Model file for the job. Use its own axes, mm. Round coordinates to 2 decimals unless told otherwise and drop trailing zeros. Write each loop counter-clockwise with the first axis right and the second up, starting at its lowest first coordinate (ties: lowest second). Pieces come first, ordered by that corner, then holes. Notation, with made-up numbers: (-10, 21) - (35, 21) arc R24 cw to (35, 43) - close; hole circle Ø5 at (60, -28). An arc over 180 degrees is marked (long way). One line per item, written item: value.
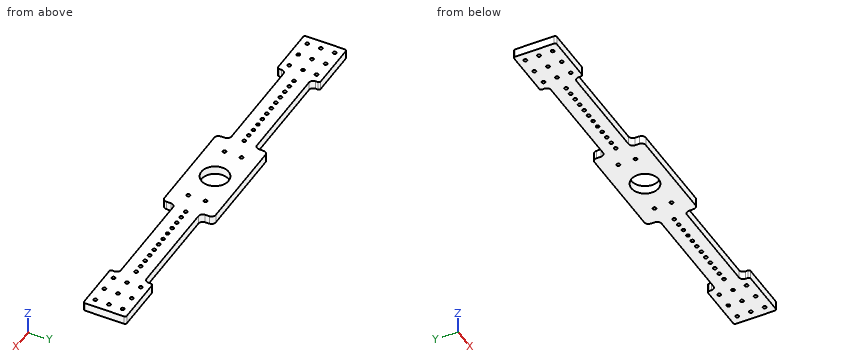
from build123d import *

# Parameters (mm, degrees)
BOSS_EXTRUDE1_DEPTH = 10
SKETCH2_R           = 2
SKETCH2_R_2         = 16
CUT_EXTRUDE1_DEPTH  = 11
FILLET1_R           = 5
SKETCH3_R           = 2
CUT_EXTRUDE2_DEPTH  = 11
SKETCH4_R           = 2
CUT_EXTRUDE3_DEPTH  = 11
LPATTERN1_COUNT     = 6
LPATTERN1_PITCH     = 10
LPATTERN1_COL_COUNT = 6
LPATTERN1_COL_PITCH = 10
SKETCH5_R           = 2
CUT_EXTRUDE4_DEPTH  = 11
FILLET2_R           = 2


with BuildPart() as part:
    # Sketch1 → Boss-Extrude1 (new body)
    with BuildSketch(Plane.XY):
        Polygon((245, 5), (245, 55), (185, 55), (185, 45), (60, 45), (60, 60), (-60, 60), (-60, 45), (-185, 45), (-185, 55), (-245, 55), (-245, 5), (-185, 5), (-185, 15), (-60, 15), (-60, 0), (60, 0), (60, 15), (185, 15), (185, 5), align=None)
    extrude(amount=BOSS_EXTRUDE1_DEPTH)

    # Sketch2 → Cut-Extrude1 (cut, through all)
    with BuildSketch(Plane.XY.offset(10)):
        with Locations((40, 20)):
            Circle(SKETCH2_R)
        with Locations((40, 40)):
            Circle(SKETCH2_R)
        with Locations((-40, 40)):
            Circle(SKETCH2_R)
        with Locations((-40, 20)):
            Circle(SKETCH2_R)
        with Locations((0, 30)):
            Circle(SKETCH2_R_2)
    extrude(amount=-CUT_EXTRUDE1_DEPTH, mode=Mode.SUBTRACT)

    # Fillet1
    fillet1_edges = [part.edges().sort_by_distance(p)[0] for p in [
        (185, 15, 5),
        (60, 15, 5),
        (60, 0, 5),
        (-60, 0, 5),
        (-60, 15, 5),
        (-185, 15, 5),
        (-185, 45, 5),
        (-60, 45, 5),
        (-60, 60, 5),
        (60, 60, 5),
        (60, 45, 5),
        (185, 45, 5),
    ]]
    fillet(fillet1_edges, radius=FILLET1_R)

    # Sketch3 → Cut-Extrude2 (cut, through all)
    with BuildSketch(Plane.XY.offset(10)):
        with Locations((-125, 30)):
            Circle(SKETCH3_R)
        with Locations((125, 30)):
            Circle(SKETCH3_R)
    cut_extrude2 = extrude(amount=-CUT_EXTRUDE2_DEPTH, mode=Mode.SUBTRACT)

    # Sketch4 → Cut-Extrude3 (cut, through all)
    with BuildSketch(Plane.XY.offset(10)):
        with Locations((-235, 14)):
            Circle(SKETCH4_R)
        with Locations((-215, 14)):
            Circle(SKETCH4_R)
        with Locations((-195, 14)):
            Circle(SKETCH4_R)
        with Locations((-195, 46)):
            Circle(SKETCH4_R)
        with Locations((-215, 46)):
            Circle(SKETCH4_R)
        with Locations((-235, 46)):
            Circle(SKETCH4_R)
        with Locations((235, 46)):
            Circle(SKETCH4_R)
        with Locations((215, 46)):
            Circle(SKETCH4_R)
        with Locations((195, 46)):
            Circle(SKETCH4_R)
        with Locations((195, 14)):
            Circle(SKETCH4_R)
        with Locations((215, 14)):
            Circle(SKETCH4_R)
        with Locations((235, 14)):
            Circle(SKETCH4_R)
        with Locations((-235, 30)):
            Circle(SKETCH4_R)
        with Locations((-215, 30)):
            Circle(SKETCH4_R)
        with Locations((-195, 30)):
            Circle(SKETCH4_R)
        with Locations((215, 30)):
            Circle(SKETCH4_R)
        with Locations((235, 30)):
            Circle(SKETCH4_R)
        with Locations((195, 30)):
            Circle(SKETCH4_R)
    extrude(amount=-CUT_EXTRUDE3_DEPTH, mode=Mode.SUBTRACT)

    # LPattern1: Cut-Extrude2 ×6
    with Locations(*[(-i * LPATTERN1_PITCH, 0, 0) for i in range(1, LPATTERN1_COUNT)]):
        add(cut_extrude2, mode=Mode.SUBTRACT)

    # LPattern1 col: Cut-Extrude2 ×6
    with Locations(*[(i * LPATTERN1_COL_PITCH, 0, 0) for i in range(1, LPATTERN1_COL_COUNT)]):
        add(cut_extrude2, mode=Mode.SUBTRACT)

    # Sketch5 → Cut-Extrude4 (cut, through all)
    with BuildSketch(Plane.XY.offset(10)):
        with Locations((-65, 30)):
            Circle(SKETCH5_R)
        with Locations((65, 30)):
            Circle(SKETCH5_R)
    extrude(amount=-CUT_EXTRUDE4_DEPTH, mode=Mode.SUBTRACT)

    # Fillet2
    fillet2_edges = [part.edges().sort_by_distance(p)[0] for p in [
        (245, 55, 5),
        (245, 5, 5),
        (185, 5, 5),
        (-185, 5, 5),
        (-245, 5, 5),
        (-245, 55, 5),
        (-185, 55, 5),
        (185, 55, 5),
    ]]
    fillet(fillet2_edges, radius=FILLET2_R)


solid = part.part
1. Band-saw the part on A-A on x = 0. Write the cut outline in (y, z).
Report:
outline: (0, 0) - (14, 0) - (14, 10) - (0, 10) - close; (46, 0) - (60, 0) - (60, 10) - (46, 10) - close
2. Drop flat-ended pins along their axis: pin 1 (3.5 mm diameter, centred on x = 195, y = 46, fed in from +Z); pin 2 (12 mm diameter, centred on x = 7.5, y = 53, fed in from -Z); pin 3 (5 mm diameter, centred on x = 102.5, z = 4.5, fed in from -Y). Give the stop position or say it passes through.
Report:
pin 1: through
pin 2: z = 0
pin 3: y = 15
3. Wall check: probe 1 along X at (y, z) = (51.5, 2); probe 2 along Y at (x, z) = (215, 7.5); probe 3 along Y at (x, z) = (-40, 6). Give the ranges that are in metal, low to high. Write a range as [from, to].
Report:
probe 1: [-245, -185], [-60, 60], [185, 245]
probe 2: [5, 12], [16, 28], [32, 44], [48, 55]
probe 3: [0, 18], [22, 38], [42, 60]
4. Band-saw the part on B-B on z = 1.5. State how many separate pieces and enclosed holes the cut face has, plus the area to 3 significant figures.
Report:
separate pieces: 1
enclosed holes: 47
area: 19,300 mm²
